Input: part model. Units: mm. Frame: model coordinates. A direction names the side the tool comes from. Round coordinates to 2 decimals unless told otherwise and drop trailing zeros. Loops run counter-clockwise (first coordinate to the right, second up) from the corner with the lowest first, then second, coordinate; pieces in that order, holes last. Notation, with made-up numbers: (6.25, 3) - (31.25, 3) arc R12 ccw to (31.25, 18) - close; hole circle Ø1 at (47, -30). An arc over 180 degrees is marked (long way). One line per question, with ' | ' between items. Start each with the question number.
from build123d import *

# Parameters (mm, degrees)
SKETCH3_R           = 6
BOSS_EXTRUDE1_DEPTH = 10
SKETCH4_W           = 50
SKETCH4_H           = 72
BOSS_EXTRUDE2_DEPTH = 3
CUT_EXTRUDE1_DEPTH  = 95.620293806


with BuildPart() as part:
    # Sketch3 → Boss-Extrude1 (new body)
    with BuildSketch(Plane(origin=(0, 0, 0), x_dir=(1, 0, 0), z_dir=(0, 1, 0))):
        with BuildLine():
            Line((48, -36), (-48, -36))
            ThreePointArc((-48, -36), (-56.485281374, -32.485281374), (-60, -24))
            Line((-60, -24), (-60, 24))
            ThreePointArc((-60, 24), (-56.485281374, 32.485281374), (-48, 36))
            Line((-48, 36), (48, 36))
            ThreePointArc((48, 36), (56.485281374, 32.485281374), (60, 24))
            Line((60, 24), (60, -24))
            ThreePointArc((60, -24), (56.485281374, -32.485281374), (48, -36))
        make_face()
        with Locations(Location((-48, 24, 0), (0, 0, 270))):
            Circle(SKETCH3_R, mode=Mode.SUBTRACT)
        with Locations(Location((-48, -24, 0), (0, 0, 270))):
            Circle(SKETCH3_R, mode=Mode.SUBTRACT)
        with Locations(Location((48, -24, 0), (0, 0, 270))):
            Circle(SKETCH3_R, mode=Mode.SUBTRACT)
        with Locations(Location((48, 24, 0), (0, 0, 270))):
            Circle(SKETCH3_R, mode=Mode.SUBTRACT)
    extrude(amount=BOSS_EXTRUDE1_DEPTH)

    # Sketch4 → Boss-Extrude2 (add)
    with BuildSketch(Plane(origin=(0, 10, 0), x_dir=(1, 0, 0), z_dir=(0, 1, 0))):
        Rectangle(SKETCH4_W, SKETCH4_H)
    extrude(amount=BOSS_EXTRUDE2_DEPTH)

    # Sketch5 → Cut-Extrude1 (cut, through all)
    with BuildSketch(Plane.XY.offset(36)):
        Polygon((0, 0), (28, 0), (25, 3), (-25, 3), (-28, 0), align=None)
    extrude(amount=-CUT_EXTRUDE1_DEPTH, mode=Mode.SUBTRACT)


solid = part.part
(1) Section B-B, the plane x = -51.5. Output: boundary loops of the cut face in (y, z).
(2) Line query: line 1 along X through (y, z) = (8, 24); line 2 along Z through (x, y) = (-52, 3.25); line 3 along Y through (x, z) = (48, -9). Output: solid intervals per line, ascending. Write a range as from..to.
(3) Pull-direction query (Z, two-part tool) for faces 5 (the face through (-25, 11, 1)), 6 (the face through (1, 6, 36)), 7 (the face through (-48, 5, 18)); classes: released by +Z, released by -Z, zero draft, split by the parting line, or undercut.
(4) Section A-A, the plane z = 4.5. Output: boundary loops of the cut face in (x, y).
(5) Pin query (flat end, axial travel): P1, Ø14, axis at x = -48, z = 24, coming from the +Y side; P2, Ø2.5, axis at y = 11.5, z = -10.5, coming from the -X side; P3, Ø0.9, axis at y = 11.5, z = -17, coming from the +X side. Return the tip coordinate at first contact, or that it passes through.
(6) Section D-D, the plane x = -12.5. Output: boundary loops of the cut face in (y, z), plus the area to 3 significant figures.
(7) Section C-C, the plane z = 20. Output: boundary loops of the cut face in (x, y), plus the area to 3 significant figures.
(8) Reachability of faces 1 (the face through (-42, 10, -1)), 2 (the face through (-60, 5, 0)), 3 (the face through (43, 10, -1)), 4 (the face through (-26, 2, 1)) from +Z, -Z, +X, -X, +Y, -Y: full face, straight path, thin tool, end or side. Return the list, or none.
Derived:
1) outline: (0, -35.48) - (10, -35.48) - (10, -28.87) - (0, -28.87) - close; (0, -19.13) - (10, -19.13) - (10, 19.13) - (0, 19.13) - close; (0, 28.87) - (10, 28.87) - (10, 35.48) - (0, 35.48) - close
2) line 1: x = -60..-54, -42..42, 54..60 | line 2: z = -35.31..-28.47, -19.53..19.53, 28.47..35.31 | line 3: y = 0..10
3) face 5: zero draft | face 6: released by +Z | face 7: undercut
4) outline: (-60, 0) - (-28, 0) - (-25, 3) - (25, 3) - (28, 0) - (60, 0) - (60, 10) - (25, 10) - (25, 13) - (-25, 13) - (-25, 10) - (-60, 10) - close
5) P1: stops at y = 10 | P2: stops at x = -25 | P3: stops at x = 25
6) outline: (3, -36) - (13, -36) - (13, 36) - (3, 36) - close | area: 720 mm²
7) outline: (-60, 0) - (-52.47, 0) - (-52.47, 10) - (-60, 10) - close; (-43.53, 0) - (-28, 0) - (-25, 3) - (25, 3) - (28, 0) - (43.53, 0) - (43.53, 10) - (25, 10) - (25, 13) - (-25, 13) - (-25, 10) - (-43.53, 10) - close; (52.47, 0) - (60, 0) - (60, 10) - (52.47, 10) - close | area: 1,010 mm²
8) face 1: +Z, -Z, -X, +Y | face 2: +Z, -Z, -X, +Y, -Y | face 3: +Z, -Z, +X, +Y | face 4: +Z, -Z, -Y
